Input: part model. Units: mm. Frame: model coordinates. Give positions to 0.01 mm unless a question says otherwise; leave off trailing zeros. Loops run counter-clockwise (first coordinate to the right, second up) from the corner with the lowest first, then second, coordinate; pieces in that order, holes last. Notation, with made-up numbers: (13.25, 82.25) -> (52.25, 82.25) arc R13 cw to (52.25, 104.25) -> close; hole circle Ø11 at (10.5, 17). An arc over 180 degrees is marked (long way). Use CSV: the item, a comma, the result in double quotes.
```python
from build123d import *

# Parameters (mm, degrees)
SKETCH1_W           = 345
SKETCH1_H           = 750
SKETCH1_R           = 2.1
SKETCH1_W_2         = 260
SKETCH1_H_2         = 570
SKETCH1_W_3         = 12.5
SKETCH1_H_3         = 12.5
BOSS_EXTRUDE1_DEPTH = 1
SKETCH2_R           = 1.6
CUT_EXTRUDE1_DEPTH  = 1
SKETCH3_R           = 1.6
CUT_EXTRUDE2_DEPTH  = 1


with BuildPart() as part:
    # Sketch1 → Boss-Extrude1 (new body)
    with BuildSketch(Plane.XY):
        with Locations((-501.064232917, -457.603531907)):
            Rectangle(SKETCH1_W, SKETCH1_H)
        with Locations((-501.064232917, -90.603531907)):
            Circle(SKETCH1_R, mode=Mode.SUBTRACT)
        with Locations((-616.064232917, -90.603531907)):
            Circle(SKETCH1_R, mode=Mode.SUBTRACT)
        with Locations((-386.064232917, -90.603531907)):
            Circle(SKETCH1_R, mode=Mode.SUBTRACT)
        with Locations((-616.01978091, -720.603531907)):
            Circle(SKETCH1_R, mode=Mode.SUBTRACT)
        with Locations((-501.01978091, -720.603531907)):
            Circle(SKETCH1_R, mode=Mode.SUBTRACT)
        with Locations((-386.01978091, -720.603531907)):
            Circle(SKETCH1_R, mode=Mode.SUBTRACT)
        with Locations((-386.064232917, -824.603531907)):
            Circle(SKETCH1_R, mode=Mode.SUBTRACT)
        with Locations((-501.064232917, -824.603531907)):
            Circle(SKETCH1_R, mode=Mode.SUBTRACT)
        with Locations((-616.064232917, -824.603531907)):
            Circle(SKETCH1_R, mode=Mode.SUBTRACT)
        with Locations((-501.01978091, -427.603531907)):
            Rectangle(SKETCH1_W_2, SKETCH1_H_2, mode=Mode.SUBTRACT)
        with Locations((-427.16978091, -774.653531907)):
            Rectangle(SKETCH1_W_3, SKETCH1_H_3, mode=Mode.SUBTRACT)
    extrude(amount=BOSS_EXTRUDE1_DEPTH)

    # Sketch2 → Cut-Extrude1 (cut)
    with BuildSketch(Plane.XY.offset(1)):
        with Locations((-669.634232917, -97.603531907)):
            Circle(SKETCH2_R)
        with Locations((-669.634232917, -817.603531907)):
            Circle(SKETCH2_R)
        with Locations((-669.634232917, -757.603531907)):
            Circle(SKETCH2_R)
        with Locations((-669.634232917, -697.603531907)):
            Circle(SKETCH2_R)
        with Locations((-669.634232917, -637.603531907)):
            Circle(SKETCH2_R)
        with Locations((-669.634232917, -577.603531907)):
            Circle(SKETCH2_R)
        with Locations((-669.634232917, -517.603531907)):
            Circle(SKETCH2_R)
        with Locations((-669.634232917, -457.603531907)):
            Circle(SKETCH2_R)
        with Locations((-669.634232917, -397.603531907)):
            Circle(SKETCH2_R)
        with Locations((-669.634232917, -337.603531907)):
            Circle(SKETCH2_R)
        with Locations((-669.634232917, -277.603531907)):
            Circle(SKETCH2_R)
        with Locations((-669.634232917, -217.603531907)):
            Circle(SKETCH2_R)
        with Locations((-669.634232917, -157.603531907)):
            Circle(SKETCH2_R)
    extrude(amount=-CUT_EXTRUDE1_DEPTH, mode=Mode.SUBTRACT)

    # Sketch3 → Cut-Extrude2 (cut)
    with BuildSketch(Plane.XY.offset(1)):
        with Locations((-332.514232917, -97.603531907)):
            Circle(SKETCH3_R)
        with Locations((-332.514232917, -817.603531907)):
            Circle(SKETCH3_R)
        with Locations((-332.514232917, -757.603531907)):
            Circle(SKETCH3_R)
        with Locations((-332.514232917, -697.603531907)):
            Circle(SKETCH3_R)
        with Locations((-332.514232917, -637.603531907)):
            Circle(SKETCH3_R)
        with Locations((-332.514232917, -577.603531907)):
            Circle(SKETCH3_R)
        with Locations((-332.514232917, -517.603531907)):
            Circle(SKETCH3_R)
        with Locations((-332.514232917, -457.603531907)):
            Circle(SKETCH3_R)
        with Locations((-332.514232917, -397.603531907)):
            Circle(SKETCH3_R)
        with Locations((-332.514232917, -337.603531907)):
            Circle(SKETCH3_R)
        with Locations((-332.514232917, -277.603531907)):
            Circle(SKETCH3_R)
        with Locations((-332.514232917, -217.603531907)):
            Circle(SKETCH3_R)
        with Locations((-332.514232917, -157.603531907)):
            Circle(SKETCH3_R)
    extrude(amount=-CUT_EXTRUDE2_DEPTH, mode=Mode.SUBTRACT)


solid = part.part
```
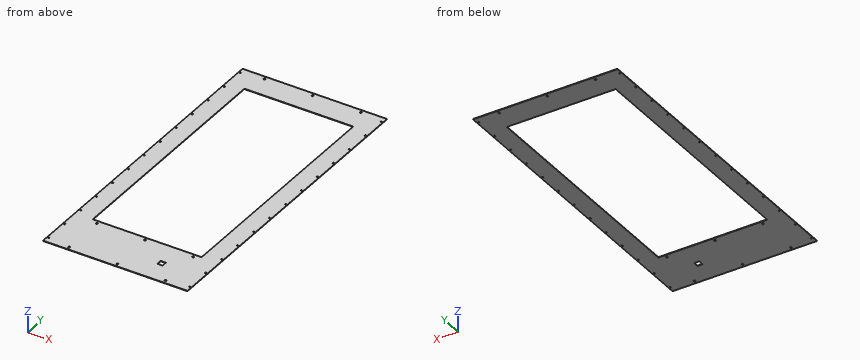
1) Ray query, line 1 (X direction, y = -251, z = 0.65); line 2 (Y direction, x = -518, z = 0.1); line 3 (X direction, y = -778, z = 0.6). Return the intervals inside material, ascending.
From the geometry:
line 1,"x = -673.56 to -631.02, -371.02 to -328.56"
line 2,"y = -832.6 to -712.6, -142.6 to -82.6"
line 3,"x = -673.56 to -433.42, -420.92 to -328.56"
2) Section query B-B (y = -566.5). Return loops of the section in (x, z), then the cut area to 3 significant figures.
From the geometry:
outline,"(-673.56, 0) -> (-631.02, 0) -> (-631.02, 1) -> (-673.56, 1) -> close; (-371.02, 0) -> (-328.56, 0) -> (-328.56, 1) -> (-371.02, 1) -> close"
area,"85.0 mm^2"
3) Section query A-A (x = -464.5). Return loops of the section in (y, z).
From the geometry:
outline,"(-832.6, 0) -> (-712.6, 0) -> (-712.6, 1) -> (-832.6, 1) -> close; (-142.6, 0) -> (-82.6, 0) -> (-82.6, 1) -> (-142.6, 1) -> close"
4) Section query C-C (z = 0.65). Give the number of separate pieces and of enclosed holes in the cut face, then the cut area to 3 significant figures.
From the geometry:
separate pieces,"1"
enclosed holes,"37"
area,"110,000 mm^2"
5) Contact query for flat-ended pins moving along their axis: pin 1 (3.5 mm diameter, centred on x = -332.51, y = -577.6, fed in from +Z); pin 2 (4 mm diameter, centred on x = -501.06, y = -824.6, fed in from +Z). Output: stop coordinate, or through.
From the geometry:
pin 1,"stops at z = 1"
pin 2,"passes through"
